```python
from build123d import *

# Parameters (mm, degrees)
F1_DEPTH      = 11.25
F1_DEPTH_BACK = 11.25
F2_R          = 7.49999
F3_W          = 5.6993120345
F3_H          = 2.3895553061
F6_DEPTH      = 2
F7_DEPTH      = 2
F8_DEPTH      = 2


# Not quite as in the source:
# - a fillet or chamfer is up to 0.001 mm smaller than in the source, because OpenCascade refuses the exact size


with BuildPart() as f1:
    # F0 (on Front) → F1 (new body, two sides)
    with BuildSketch(Plane.XZ) as f1_sk:
        Polygon((7.5, -12.9903810568), (7.5, 12.9903810568), (-15, 0), align=None)
    extrude(amount=F1_DEPTH)
    extrude(f1_sk.sketch, amount=-F1_DEPTH_BACK)

    # F2 (radius 7.5 in the source; OpenCascade refuses exactly that, so slightly less here)
    f2_edges = [f1.edges().sort_by_distance(p)[0] for p in [
        (7.5, 11.25, 0),
        (-3.75, 11.25, 6.495191),
        (-3.75, 11.25, -6.495191),
        (7.5, -11.25, 0),
        (-3.75, -11.25, 6.495191),
        (-3.75, -11.25, -6.495191),
    ]]
    fillet(f2_edges, radius=F2_R)

    # F3 (on face) → F6 (cut)
    with BuildSketch(Plane(origin=(-3.75, 0, -6.4951905284), x_dir=(0.8660254038, 0, -0.5), z_dir=(-0.5, 0, -0.8660254038))):
        with Locations((2.8496560172, 1.562116124)):
            Rectangle(F3_W, F3_H)
        with BuildLine():
            Line((-0.8410443106, 0.367338471), (0, 0.367338471))
            Line((0, 0.367338471), (0, 2.7568937771))
            Line((0, 2.7568937771), (-5.6028393047, 2.7568937771))
            Line((-5.6028393047, 2.7568937771), (-5.6028393047, 0.7928079458))
            Line((-5.6028393047, 0.7928079458), (-2.7037100927, -2.8484191874))
            Line((-2.7037100927, -2.8484191874), (-1.2665137854, -1.6956937498))
            Line((-1.2665137854, -1.6956937498), (-2.3103981945, -0.3970223878))
            add(Edge.make_bspline(
                [(-3.0896010117, 0.4291799644), (-2.4959226748, -0.1644983725), (-2.3103981945, -0.3970223878)],
                knots=[0, 0, 0, 1, 1, 1], degree=2))
            Line((-3.0896010117, 0.4291799644), (-1.9146126366, 0.3920750683))
            Line((-1.9146126366, 0.3920750683), (-0.8410443106, 0.367338471))
        make_face()
    extrude(amount=-F6_DEPTH, mode=Mode.SUBTRACT)

    # F4 (on face) → F7 (cut)
    with BuildSketch(Plane.YZ.offset(7.5)):
        with BuildLine():
            add(Edge.make_bspline(
                [(0.1534139825, 0), (-0.1261569639, -0.3061831776), (-0.2635343428, -0.4836289588)],
                knots=[0.5438727063, 0.5438727063, 0.5438727063, 1, 1, 1], degree=2))
            Line((0.1534139825, 0), (-1.9043553856, 0))
            add(Edge.make_bspline(
                [(-2.4683418116, -0.9662925903), (-2.2786358022, -0.49373663), (-1.9043553856, 0)],
                knots=[0, 0, 0, 0.8852247383, 0.8852247383, 0.8852247383], degree=2))
            add(Edge.make_bspline(
                [(-2.682644464, -2.110205397), (-2.682644464, -1.5001185668), (-2.4683418116, -0.9662925903)],
                knots=[0, 0, 0, 1, 1, 1], degree=2))
            add(Edge.make_bspline(
                [(-2.3322306675, -3.3525815846), (-2.682644464, -2.8091023355), (-2.682644464, -2.110205397)],
                knots=[0, 0, 0, 1, 1, 1], degree=2))
            add(Edge.make_bspline(
                [(-1.3485621865, -4.1972429397), (-1.981816871, -3.8960608337), (-2.3322306675, -3.3525815846)],
                knots=[0, 0, 0, 1, 1, 1], degree=2))
            add(Edge.make_bspline(
                [(0.1110126353, -4.4984250458), (-0.7153075019, -4.4984250458), (-1.3485621865, -4.1972429397)],
                knots=[0, 0, 0, 1, 1, 1], degree=2))
            add(Edge.make_bspline(
                [(1.2452721693, -4.3748631562), (0.7384753562, -4.4984250458), (0.1110126353, -4.4984250458)],
                knots=[0, 0, 0, 1, 1, 1], degree=2))
            add(Edge.make_bspline(
                [(2.1806742872, -4.0225187051), (1.7520689824, -4.2513012665), (1.2452721693, -4.3748631562)],
                knots=[0, 0, 0, 1, 1, 1], degree=2))
            add(Edge.make_bspline(
                [(3.2599101673, -3.2377076403), (2.609279592, -3.7937361438), (2.1806742872, -4.0225187051)],
                knots=[0, 0, 0, 1, 1, 1], degree=2))
            Line((3.2599101673, -3.2377076403), (2.2463165411, -2.036840525))
            add(Edge.make_bspline(
                [(1.2385148785, -2.7067776456), (1.72117851, -2.4712377934), (2.2463165411, -2.036840525)],
                knots=[0, 0, 0, 1, 1, 1], degree=2))
            add(Edge.make_bspline(
                [(0.2442277976, -2.9423174978), (0.755851247, -2.9423174978), (1.2385148785, -2.7067776456)],
                knots=[0, 0, 0, 1, 1, 1], degree=2))
            add(Edge.make_bspline(
                [(-0.5376872855, -2.682644464), (-0.2442277976, -2.9423174978), (0.2442277976, -2.9423174978)],
                knots=[0, 0, 0, 1, 1, 1], degree=2))
            add(Edge.make_bspline(
                [(-0.8311467735, -1.8920414356), (-0.8311467735, -2.4229714303), (-0.5376872855, -2.682644464)],
                knots=[0, 0, 0, 1, 1, 1], degree=2))
            add(Edge.make_bspline(
                [(-0.6979316112, -1.2047284243), (-0.8311467735, -1.5368010028), (-0.8311467735, -1.8920414356)],
                knots=[0, 0, 0, 1, 1, 1], degree=2))
            add(Edge.make_bspline(
                [(-0.2635343428, -0.4836289588), (-0.5647164489, -0.8726558458), (-0.6979316112, -1.2047284243)],
                knots=[0, 0, 0, 1, 1, 1], degree=2))
        make_face()
        with BuildLine():
            Line((-1.9043553856, 0), (0.1534139825, 0))
            add(Edge.make_bspline(
                [(1.0222815716, 0.9131995908), (0.4867661175, 0.3650837732), (0.1534139825, 0)],
                knots=[0, 0, 0, 0.5438727063, 0.5438727063, 0.5438727063], degree=2))
            Line((1.0222815716, 0.9131995908), (3.236742313, 3.1508281866))
            Line((3.236742313, 3.1508281866), (3.236742313, 4.4482280281))
            Line((3.236742313, 4.4482280281), (-2.9297682434, 4.4482280281))
            Line((-2.9297682434, 4.4482280281), (-2.9297682434, 2.8786058984))
            Line((-2.9297682434, 2.8786058984), (0.9141649181, 2.8786058984))
            Line((0.9141649181, 2.8786058984), (0.9141649181, 2.7955877538))
            Line((0.9141649181, 2.7955877538), (-0.2210599432, 1.7279358009))
            add(Edge.make_bspline(
                [(-1.8041966546, 0.128388526), (-1.3543541501, 0.6892436658), (-0.2210599432, 1.7279358009)],
                knots=[0, 0, 0, 1, 1, 1], degree=2))
            add(Edge.make_bspline(
                [(-1.9043553856, 0), (-1.8558274458, 0.0640162305), (-1.8041966546, 0.128388526)],
                knots=[0.8852247383, 0.8852247383, 0.8852247383, 1, 1, 1], degree=2))
        make_face()
    extrude(amount=-F7_DEPTH, mode=Mode.SUBTRACT)

    # F5 (on face) → F8 (cut)
    with BuildSketch(Plane(origin=(-3.75, 0, 6.4951905284), x_dir=(0.8660254038, 0, 0.5), z_dir=(-0.5, 0, 0.8660254038))):
        with BuildLine():
            Line((0.8145773358, 1.8911934049), (0, 1.8911934049))
            Line((0, 1.8911934049), (0, 0))
            Line((0, 0), (0, -1.5006215977))
            add(Edge.make_bspline(
                [(0.1648783041, -0.7331196022), (0.1120638425, -1.1571661487), (0, -1.5006215977)],
                knots=[0, 0, 0, 0.3899595317, 0.3899595317, 0.3899595317], degree=2))
            Line((0.1648783041, -0.7331196022), (0.2002093693, -0.7331196022))
            add(Edge.make_bspline(
                [(1.0108610311, -2.163046323), (0.422009945, -1.6536901335), (0.2002093693, -0.7331196022)],
                knots=[0, 0, 0, 1, 1, 1], degree=2))
            add(Edge.make_bspline(
                [(2.4398063334, -2.6724025124), (1.5997121172, -2.6724025124), (1.0108610311, -2.163046323)],
                knots=[0, 0, 0, 1, 1, 1], degree=2))
            add(Edge.make_bspline(
                [(4.0090944779, -1.8656765245), (3.4447788537, -2.6724025124), (2.4398063334, -2.6724025124)],
                knots=[0, 0, 0, 1, 1, 1], degree=2))
            add(Edge.make_bspline(
                [(4.5734101021, 0.3327008636), (4.5734101021, -1.0589505365), (4.0090944779, -1.8656765245)],
                knots=[0, 0, 0, 1, 1, 1], degree=2))
            add(Edge.make_bspline(
                [(3.6901334729, 3.2592907616), (4.5734101021, 2.0325176655), (4.5734101021, 0.3327008636)],
                knots=[0, 0, 0, 1, 1, 1], degree=2))
            Line((3.6901334729, 3.2592907616), (2.3848468987, 2.3819026433))
            add(Edge.make_bspline(
                [(2.8932216697, 1.3671159382), (2.7460088982, 1.8244569484), (2.3848468987, 2.3819026433)],
                knots=[0, 0, 0, 1, 1, 1], degree=2))
            add(Edge.make_bspline(
                [(3.0404344412, 0.4681366135), (3.0404344412, 0.909774928), (2.8932216697, 1.3671159382)],
                knots=[0, 0, 0, 1, 1, 1], degree=2))
            add(Edge.make_bspline(
                [(2.0217220623, -0.8077074064), (3.0404344412, -0.8077074064), (3.0404344412, 0.4681366135)],
                knots=[0, 0, 0, 1, 1, 1], degree=2))
            add(Edge.make_bspline(
                [(1.0874116723, -0.3258309343), (1.3602460089, -0.8077074064), (2.0217220623, -0.8077074064)],
                knots=[0, 0, 0, 1, 1, 1], degree=2))
            add(Edge.make_bspline(
                [(0.8145773358, 1.1983119602), (0.8145773358, 0.1560455378), (1.0874116723, -0.3258309343)],
                knots=[0, 0, 0, 1, 1, 1], degree=2))
            Line((0.8145773358, 1.1983119602), (0.8145773358, 1.8911934049))
        make_face()
        with BuildLine():
            Line((0, 0), (0, 1.8911934049))
            Line((0, 1.8911934049), (-0.6398848469, 1.8911934049))
            Line((-0.6398848469, 1.8911934049), (-0.6398848469, 1.2100889819))
            add(Edge.make_bspline(
                [(-0.9038864172, -0.4337869668), (-0.6398848469, 0.0814577336), (-0.6398848469, 1.2100889819)],
                knots=[0, 0, 0, 1, 1, 1], degree=2))
            add(Edge.make_bspline(
                [(-1.7979586496, -0.9490316671), (-1.1678879874, -0.9490316671), (-0.9038864172, -0.4337869668)],
                knots=[0, 0, 0, 1, 1, 1], degree=2))
            add(Edge.make_bspline(
                [(-2.8235409579, -0.5015048417), (-2.5045799529, -0.9490316671), (-1.7979586496, -0.9490316671)],
                knots=[0, 0, 0, 1, 1, 1], degree=2))
            add(Edge.make_bspline(
                [(-3.1425019628, 0.8862208846), (-3.1425019628, -0.0539780162), (-2.8235409579, -0.5015048417)],
                knots=[0, 0, 0, 1, 1, 1], degree=2))
            add(Edge.make_bspline(
                [(-2.9766422403, 2.1247710024), (-3.1425019628, 1.4986260141), (-3.1425019628, 0.8862208846)],
                knots=[0, 0, 0, 1, 1, 1], degree=2))
            add(Edge.make_bspline(
                [(-2.5477623659, 3.2710677833), (-2.8107825177, 2.7509159906), (-2.9766422403, 2.1247710024)],
                knots=[0, 0, 0, 1, 1, 1], degree=2))
            Line((-2.5477623659, 3.2710677833), (-4.1612143418, 3.2710677833))
            add(Edge.make_bspline(
                [(-4.6460350694, 0.6820858414), (-4.6460350694, 2.1424365349), (-4.1612143418, 3.2710677833)],
                knots=[0, 0, 0, 1, 1, 1], degree=2))
            add(Edge.make_bspline(
                [(-3.9246924889, -1.9971866004), (-4.6460350694, -1.0589505365), (-4.6460350694, 0.6820858414)],
                knots=[0, 0, 0, 1, 1, 1], degree=2))
            add(Edge.make_bspline(
                [(-1.9098403559, -2.9354226642), (-3.2033499084, -2.9354226642), (-3.9246924889, -1.9971866004)],
                knots=[0, 0, 0, 1, 1, 1], degree=2))
            add(Edge.make_bspline(
                [(-0.4956163308, -2.3779769694), (-1.0206752159, -2.9354226642), (-1.9098403559, -2.9354226642)],
                knots=[0, 0, 0, 1, 1, 1], degree=2))
            add(Edge.make_bspline(
                [(0, -1.5006215977), (-0.1753091627, -2.0379125367), (-0.4956163308, -2.3779769694)],
                knots=[0.3899595317, 0.3899595317, 0.3899595317, 1, 1, 1], degree=2))
            Line((0, -1.5006215977), (0, 0))
        make_face()
    extrude(amount=-F8_DEPTH, mode=Mode.SUBTRACT)


solid = f1.part
```
The model under review builds one solid part; all positions refer to its coordinate system, in mm. A direction names the side the tool comes from. Round coordinates to 2 decimals unless told otherwise and drop trailing zeros. Order: outer loops, then holes, each group sorted by start corner. A loop starts at its lowest first (then second) coordinate and runs counter-clockwise, first axis right, second up. Notation, with made-up numbers: M 85,46.5 L 97,46.5 A32 cw 97,82.5 Z; hole C 60.5,69 d5. An arc over 180 degrees is marked long. Use a Markdown table: item, result.
1) Insertion check: pin 1 (10 mm diameter, centred on x = -1, z = 2, fed in from -Y); pin 2 (3 mm diameter, centred on y = -6.5, z = 3.5, fed in from +X); pin 3 (1 mm diameter, centred on x = 0.5, y = -2.5, fed in from +Z); pin 4 (1.4 mm diameter, centred on x = 7, z = 4, fed in from -Y). Each pin has a flat end and moves straight along its axis. Give the tip position at first contact, or say it passes through.
Report:
| item | result |
|---|---|
| pin 1 | y = -11.25 |
| pin 2 | x = 7.4 |
| pin 3 | z = 9.24 |
| pin 4 | y = -7.82 |
2) Wall thickness on line 1 along Y through (x, z) = (1, -8.5); line 2 along Y through (x, z) = (-6.5, -4); line 3 along Z through (x, y) = (1, 8.5): over which ranges is each line inside the solid? List them lowest first. Write a range as [from, to].
Report:
| item | result |
|---|---|
| line 1 | [-6.78, -2.76], [-0.37, 6.78] |
| line 2 | [-7.09, -2.76], [1.69, 7.09] |
| line 3 | [-7.28, 7.28] |
3) Tool access review of faces 1 (the face through (-2.938, 7.984, -5.452)), 2 (the face through (-0.619, 2.827, 7.165)), 3 (the face through (-8.11, -1.79, -2.84)), 4 (the face through (6.514, 2.76, -2.646)), 5 (the face through (6.191, 7.984, 0.182)): name each direction out of +Z, -Z, +X, -X, +Y, -Y from which nothing blocks a thin tool from reaching the whole face with its end or side.
Report:
| item | result |
|---|---|
| face 1 | -Z, -X, +Y |
| face 2 | none |
| face 3 | -Z |
| face 4 | +X |
| face 5 | +Z, -Z, +X, +Y |
4) Draft analysis for pull direction X (two halves, no side actions). For faces 6 (the face through (-3.592, -1.719, 6.586)), 7 (the face through (-3.8, 1.6, 5.3)), 8 (the face through (7, 3.237, 4)), state which applies: released by +X, released by -X, zero draft, split by the parting line, or undercut.
Report:
| item | result |
|---|---|
| face 6 | released by -X |
| face 7 | undercut |
| face 8 | zero draft |
5) Consider section A-A (y = 9.25). Write out the cut boundary in (x, z), then the cut area to 3 significant figures.
Report:
| item | result |
|---|---|
| outline | M -10.2,0 L 5.1,-8.83 L 5.1,8.83 Z |
| area | 135 mm^2 |
